```python
from build123d import *

# Parameters (mm, degrees)
BOSS_EXTRU_1_DEPTH      = 6.35
ESQUISSE2_R             = 1.5
ENL_V_MAT_EXTRU_1_DEPTH = 6.35
ESQUISSE3_R             = 1.5
ENL_V_MAT_EXTRU_2_DEPTH = 6.35


with BuildPart() as part:
    # Esquisse1 → Boss.-Extru.1 (new body)
    with BuildSketch(Plane.XY):
        with BuildLine():
            Line((0, 6), (101.6, 6))
            ThreePointArc((101.6, 6), (107.6, 0), (101.6, -6))
            Line((101.6, -6), (0, -6))
            ThreePointArc((0, -6), (-6, 0), (0, 6))
        make_face()
    extrude(amount=BOSS_EXTRU_1_DEPTH)

    # Esquisse2 → Enlèv. mat.-Extru.1 (cut)
    with BuildSketch(Plane.XY.offset(6.35)):
        Circle(ESQUISSE2_R)
    extrude(amount=-ENL_V_MAT_EXTRU_1_DEPTH, mode=Mode.SUBTRACT)

    # Esquisse3 → Enlèv. mat.-Extru.2 (cut)
    with BuildSketch(Plane.XY.offset(6.35)):
        with Locations((101.6, 0)):
            Circle(ESQUISSE3_R)
    extrude(amount=-ENL_V_MAT_EXTRU_2_DEPTH, mode=Mode.SUBTRACT)


solid = part.part
```
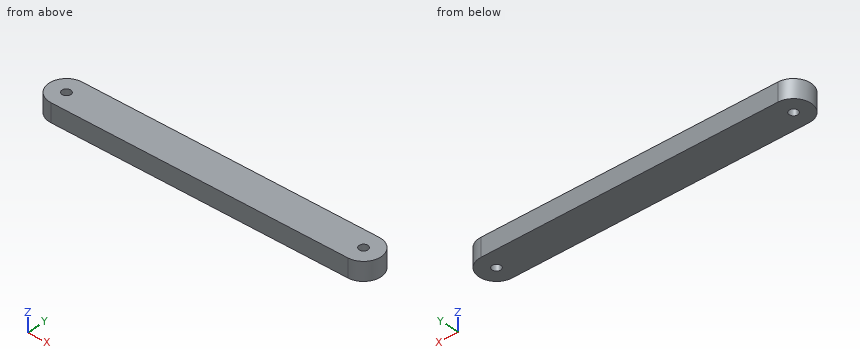
Here's how the part is built. I have some questions about the finished solid (model axes, mm). Coordinates: 2 decimals unless noted, no trailing zeros. Write each loop counter-clockwise with the first axis right and the second up, starting at its lowest first coordinate (ties: lowest second). Pieces come first, ordered by that corner, then holes. Notation, with made-up numbers: M -29,81 L 25,81 A26 ccw 25,96 Z; hole C -16,11.25 d8. An arc over 180 degrees is marked long. Answer as CSV lines item,"result". Start each with the question number.
Q1. I need wall thicknesses on probe 1 along Y at (x, z) = (101.6, 3.5); probe 2 along X at (y, z) = (-1, 2.75); probe 3 along X at (y, z) = (3.5, 0.5). Which ranges of each line are inside material? Lowest first, please. Write a range as [from, to].
Q2. Suppose I cut it at B-B, the plane z = 3. List the corners of the cut face in (x, y) for me.
Q3. Suppose I cut it at A-A, the plane y = 0. List the corners of the cut face in (x, z) for me.
Q4. Will this pin go through, and if not, where does the flat tip stop? pin 1 Ø1.5 at (y, z) = (3.5, 3.5) entering from +X.
Entries:
1,probe 1,"y = [-6, -1.5], [1.5, 6]"
1,probe 2,"x = [-5.92, -1.12], [1.12, 100.48], [102.72, 107.52]"
1,probe 3,"x = [-4.87, 106.47]"
2,outline,"M 0,-6 L 101.6,-6 A6 ccw 101.6,6 L 0,6 A6 ccw Z; hole C 0,0 d3; hole C 101.6,0 d3"
3,outline,"M -6,0 L -1.5,0 L -1.5,6.35 L -6,6.35 Z; M 1.5,0 L 100.1,0 L 100.1,6.35 L 1.5,6.35 Z; M 103.1,0 L 107.6,0 L 107.6,6.35 L 103.1,6.35 Z"
4,pin 1,"stops at x = 106.93"
